```python
from build123d import *

# Parameters (mm, degrees)
F0_R      = 1.5
F1_DEPTH  = 4
F3_DEPTH  = 2.5
F5_DEPTH  = 30
F7_DEPTH  = 5
F14_DEPTH = 5


with BuildPart() as f1:
    # F0 (on Top) → F1 (new body)
    with BuildSketch(Plane.XY):
        with BuildLine():
            Line((15, 10), (-15, 10))
            ThreePointArc((-15, 10), (-25, 0), (-15, -10))
            Line((-15, -10), (15, -10))
            ThreePointArc((15, -10), (25, 0), (15, 10))
        make_face()
        with Locations((-15, 0)):
            Circle(F0_R, mode=Mode.SUBTRACT)
        with Locations((15, 0)):
            Circle(F0_R, mode=Mode.SUBTRACT)
    extrude(amount=F1_DEPTH)

    # F2 (on Right) → F3 (join, symmetric)
    with BuildSketch(Plane.YZ):
        with BuildLine():
            Line((-10, 0), (-10, 4))
            Line((-10, 4), (-26, 4))
            add(Edge.make_bspline(
                [(-26, 4), (-26, 3), (-25.0865402228, -0.0476028537), (-20, 0), (-18, 0)],
                knots=[0, 0, 0, 0, 0.4160108935, 1, 1, 1, 1], degree=3))
            Line((-18, 0), (-10, 0))
        make_face()
    extrude(amount=F3_DEPTH, both=True)

    # F4 (on face) → F5 (join)
    with BuildSketch(Plane.XY.offset(4)):
        Polygon((-2.5, -21), (-2.5, -26), (0, -26), (2.5, -26), (2.5, -21), align=None)
    extrude(amount=F5_DEPTH)

    # F6 (on face) → F7 (cut, through all)
    with BuildSketch(Plane(origin=(-2.5, 0, 0), x_dir=(0, -1, 0), z_dir=(-1, 0, 0))):
        with BuildLine():
            add(Edge.make_bspline(
                [(26, 24.786574766), (26, 28.7767909467), (24.6865190566, 34), (21, 34)],
                knots=[0, 0, 0, 0, 10.48270979, 10.48270979, 10.48270979, 10.48270979], degree=3))
            Line((26, 24.786574766), (26, 34))
            Line((26, 34), (21, 34))
        make_face()
    extrude(amount=-F7_DEPTH, mode=Mode.SUBTRACT)

    # F9 (on plane+point) → F10 (revolve, cut)
    with BuildSketch(Plane.YZ.offset(15)):
        Polygon((3.5, 4), (0, 4), (0, 2), align=None)
    revolve(axis=Axis((15, 0, 3), (0, 0, -1)), mode=Mode.SUBTRACT)

    # F12 (on plane+point) → F13 (revolve, cut)
    with BuildSketch(Plane.YZ.offset(-15)):
        Polygon((3.5, 4), (0, 4), (0, 2), align=None)
    revolve(axis=Axis((-15, 0, 0), (0, 0, -1)), mode=Mode.SUBTRACT)

    # F6 (on face) → F14 (join, through all)
    with BuildSketch(Plane(origin=(-2.5, 0, 0), x_dir=(0, -1, 0), z_dir=(-1, 0, 0))):
        Polygon((21, 26), (21, 34), (16, 34), align=None)
    extrude(amount=-F14_DEPTH)


solid = f1.part
```
Read the model definition and answer for the solid it produces. Units are mm, in the model's axes. A direction names the side the tool comes from. Give positions to 0.01 mm unless a question says otherwise; leave off trailing zeros. Loops run counter-clockwise (first coordinate to the right, second up) from the corner with the lowest first, then second, coordinate; pieces in that order, holes last.
Item 1: Each of these flat-tipped pins is pushed along its axis until it touches: pin 1 Ø3 at (x, z) = (7.5, 3) entering from -Y; pin 2 Ø4 at (x, z) = (-0.5, 11.5) entering from +Y; pin 3 Ø17.5 at (y, z) = (-20, 19) entering from -X; pin 4 Ø3 at (x, y) = (-15, -13) entering from +Z. Where does it stop, or does it pass through?
Item 2: The part is cut by section A-A (y = 0). Write down the section's boundary in (x, z), and give its area (3 significant figures).
Item 3: The part is cut by section B-B (z = 13). Write down the section's boundary in (x, y).
Item 4: The mould has two halves that part along X. Classify faces 1 (the flat face through (-2.5, -21.4, 17.2)), 2 (the flat face through (0, -26, 14)), 3 (the cylindrical face through (13.5, 0.07, 1.41)): released by +X, released by -X, zero draft, split by the parting line, or undercut.
Item 5: The part is cut by section C-C (x = 7). Write down the section's boundary in (y, z).
Item 6: For faces 4 (the flat face through (-0.035, -18.465, 30.056)), 5 (the flat face through (-9, -10, 2)), 6 (the flat face through (0, -1, 0)), 7 (the flat face through (9, -10, 2)), determine the directions among +Z, -Z, +X, -X, +Y, -Y from which every point of the face is accessible in a straight line to the end or side of a thin tool.
Item 7: Find the intervals of material crossed by line 1 along X through (y, z) = (0, 0.65); line 2 along Y through (x, z) = (-15, 1.85); line 3 along Z through (x, y) = (-6.5, -8.5), in increasing order.
Taken from the geometry:
1. pin 1: stops at y = -10
1. pin 2: stops at y = -21
1. pin 3: stops at x = -2.5
1. pin 4: passes through
2. outline: (-25, 0) - (-16.5, 0) - (-16.5, 2.86) - (-18.5, 4) - (-25, 4) - close; (-13.5, 0) - (13.5, 0) - (13.5, 2.86) - (11.5, 4) - (-11.5, 4) - (-13.5, 2.86) - close; (16.5, 0) - (25, 0) - (25, 4) - (18.5, 4) - (16.5, 2.86) - close
2. area: 171 mm2
3. outline: (-2.5, -26) - (2.5, -26) - (2.5, -21) - (-2.5, -21) - close
4. face 1: released by -X
4. face 2: zero draft
4. face 3: undercut
5. outline: (-10, 0) - (10, 0) - (10, 4) - (-10, 4) - close
6. face 4: +X, -X, +Y
6. face 5: +Z, -Z, -X, -Y
6. face 6: -Z, +X, -X, +Y, -Y
6. face 7: +Z, -Z, +X, -Y
7. line 1: x = -25 to -16.5, -13.5 to 13.5, 16.5 to 25
7. line 2: y = -10 to -1.5, 1.5 to 10
7. line 3: z = 0 to 4
